CAD build for the part. Positions are in the model's coordinates, mm. Face numbers are marked on the shaded views. A direction names the side the tool comes from. Coordinates: 2 decimals unless noted, no trailing zeros. Loops run counter-clockwise (first coordinate to the right, second up) from the corner with the lowest first, then second, coordinate; pieces in that order, holes last.
1) Saw through at A-A, the plane z = 17. Write the cut outline in (x, y), and give its area (3 significant figures).
2) Which spindle directions (+Z, -Z, +X, -X, +Y, -Y) get a long thin tool onto all of the face, cutting with end or side? Do the marked faces 1, 2 and 3. Say none if no direction does.
3) Wall check: line 1 along Y through (x, z) = (-42, 4); line 2 along X through (y, z) = (-6.25, 20). Give the ranges that are in metal, low to high.
4) Saw through at B-B, the plane y = -1.25. Write the cut outline in (x, z), and give its area (3 significant figures).
5) Saw through at C-C, the plane x = -28.5. Write the cut outline in (y, z), and give its area (3 significant figures).
6) Pin check, flat tips, straight feed: pin 1 Ø10 at (x, z) = (-38, 4.5) entering from +Y; pin 2 Ø1.9 at (y, z) = (-22.5, 19.5) entering from +X; pin 3 Ø8 at (x, y) = (-25.5, -2.5) entering from +Z; pin 4 Ø7.5 at (x, z) = (-37, 18) entering from -Y. Stop position of each tip, or through.
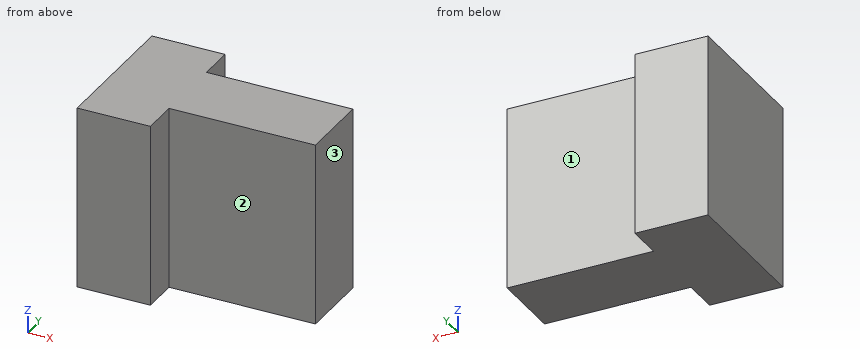
```python
from build123d import *

# Parameters (mm, degrees)
F0_W     = 38.1
F0_H     = 31.75
F1_DEPTH = 25.4
F2_W     = 25.4
F2_H     = 31.75
F3_DEPTH = 6.35
F4_W     = 25.4
F4_H     = 31.75
F5_DEPTH = 6.35


# Not quite as in the source:
# - a feature names something its author has since deleted; it is built from what else it names


with BuildPart() as f1:
    # F0 (on Front) → F1 (new body)
    with BuildSketch(Plane.XZ):
        with Locations((-37.3860847076, 16.0793865216)):
            Rectangle(F0_W, F0_H)
    extrude(amount=F1_DEPTH)

    # F2 (on face) → F3 (cut)
    with BuildSketch(Plane.XZ.offset(25.4)):
        with Locations((-31.0360847076, 16.0793865216)):
            Rectangle(F2_W, F2_H)
    extrude(amount=-F3_DEPTH, mode=Mode.SUBTRACT)

    # F4 (on face) → F5 (cut)
    with BuildSketch(Plane(origin=(0, 0, 0), x_dir=(-1, 0, 0), z_dir=(0, 1, 0))):
        with Locations((31.0360847076, 16.0793865216)):
            Rectangle(F4_W, F4_H)
    extrude(amount=-F5_DEPTH, mode=Mode.SUBTRACT)


solid = f1.part
```
Data:
1. outline: (-56.44, -25.4) - (-43.74, -25.4) - (-43.74, -19.05) - (-18.34, -19.05) - (-18.34, -6.35) - (-43.74, -6.35) - (-43.74, 0) - (-56.44, 0) - close
1. area: 645 mm2
2. face 1: +Z, -Z, +X, +Y
2. face 2: +Z, -Z, +X, -Y
2. face 3: +Z, -Z, +X, +Y, -Y
3. line 1: y = -19.05 to -6.35
3. line 2: x = -56.44 to -43.74
4. outline: (-56.44, 0.2) - (-43.74, 0.2) - (-43.74, 31.95) - (-56.44, 31.95) - close
4. area: 403 mm2
5. outline: (-19.05, 0.2) - (-6.35, 0.2) - (-6.35, 31.95) - (-19.05, 31.95) - close
5. area: 403 mm2
6. pin 1: stops at y = -6.35
6. pin 2: stops at x = -43.74
6. pin 3: stops at z = 31.95
6. pin 4: stops at y = -19.05
